Can you work these out from the model? Positions are in its coordinate system, mm. Face numbers are marked on the shaded views. Coordinates: 2 decimals unless noted, no trailing zeros. Order: outer loops, then holes, each group sorted by start corner. A loop starts at its lowest first (then second) coordinate and runs counter-clockwise, first axis right, second up. Notation, with made-up numbers: M 74,55.25 L 87,55.25 A31 ccw 87,88.25 Z; hole C -0.5,49 d1. An arc over 180 degrees is marked long. Answer as CSV lines item,"result". Start each with the question number.
1. Will these pins go through, and if not, where does the flat tip stop? pin 1 (1.6 mm diameter, centred on y = 2.54, z = 0, fed in from +X); pin 2 (10 mm diameter, centred on x = 11, y = 11, fed in from +Z); pin 3 (2 mm diameter, centred on y = 5, z = -1.5, fed in from +X).
2. If we mould it in two halves opening along X, with no side actions, what happens to the marked faces 1, 2 and 3? For each: released by +X, released by -X, zero draft, split by the parting line, or undercut.
3. I need wall thicknesses on line 1 along X through (y, z) = (8.25, 0); line 2 along Z through (x, y) = (4, 6.75). Which ranges of each line are inside material? Lowest first, please. Write a range as from..to.
4. If we section it at B-B (y = 5): List the corners of the cut face in (x, z) for me (1 decimal).
5. If we section it at A-A (x = 0): List the corners of the cut face in (y, z) for me (1 decimal).
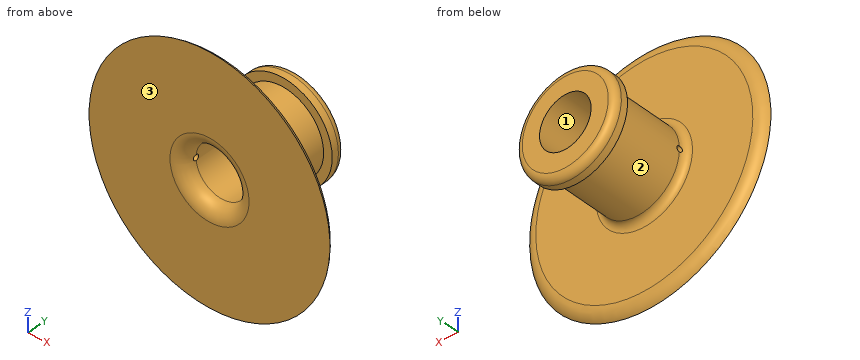
```python
from build123d import *

# Parameters (mm, degrees)
SKETCH1_R           = 22.225
BOSS_EXTRUDE1_DEPTH = 1.27
SKETCH2_R           = 7.62
BOSS_EXTRUDE2_DEPTH = 16.256
SKETCH3_R           = 4.7625
CUT_EXTRUDE1_DEPTH  = 36.986968836
FILLET1_R           = 1.27
SKETCH4_R           = 0.508
CUT_EXTRUDE2_DEPTH  = 36.986968836
FILLET2_R           = 2.54
FILLET3_R           = 2.54
SKETCH5_W           = 1.5875
SKETCH5_H           = 2.54
FILLET4_R           = 1.27


with BuildPart() as part:
    # Sketch1 → Boss-Extrude1 (new body)
    with BuildSketch(Plane(origin=(0, 0, 0), x_dir=(1, 0, 0), z_dir=(0, 1, 0))):
        with Locations(Location((0, 0, 0), (0, 0, 270))):
            Circle(SKETCH1_R)
    extrude(amount=BOSS_EXTRUDE1_DEPTH)

    # Sketch2 → Boss-Extrude2 (add)
    with BuildSketch(Plane(origin=(0, 1.27, 0), x_dir=(1, 0, 0), z_dir=(0, 1, 0))):
        with Locations(Location((0, 0, 0), (0, 0, 270))):
            Circle(SKETCH2_R)
    extrude(amount=BOSS_EXTRUDE2_DEPTH)

    # Sketch3 → Cut-Extrude1 (cut, through all)
    with BuildSketch(Plane(origin=(0, 17.526, 0), x_dir=(1, 0, 0), z_dir=(0, 1, 0))):
        with Locations(Location((0, 0, 0), (0, 0, 270))):
            Circle(SKETCH3_R)
    extrude(amount=-CUT_EXTRUDE1_DEPTH, mode=Mode.SUBTRACT)

    # Fillet1
    fillet1_edges = [part.edges().sort_by_distance(p)[0] for p in [
        (0, 1.27, -7.62),
    ]]
    fillet(fillet1_edges, radius=FILLET1_R)

    # Sketch4 → Cut-Extrude2 (cut, through all)
    with BuildSketch(Plane(origin=(0, 0, 0), x_dir=(0, 0, -1), z_dir=(1, 0, 0))):
        with Locations((0, 2.54)):
            Circle(SKETCH4_R)
    extrude(amount=-CUT_EXTRUDE2_DEPTH, mode=Mode.SUBTRACT)

    # Fillet2
    # the kernel refuses this fillet: 2.54 mm, written as the material it takes off along each edge
    with BuildSketch(Plane(origin=(0, 1.27, 0), x_dir=(0, 0, 1), z_dir=(-1, 0, 0))) as fillet2_piece_1:
        with BuildLine():
            CenterArc((20.025295474, -2.54), FILLET2_R, 30, 60)
            Line((22.225, -1.27), (22.268994091, -1.2446))
            ThreePointArc((22.268994091, -1.2446), (22.2758, -0.635), (22.2758, 0))
            Line((22.2758, 0), (22.225, 0.0508))
            Line((22.225, 0.0508), (20.025295474, 0.0508))
            Line((20.025295474, 0.0508), (20.025295474, 0))
        make_face()
    revolve(axis=Axis((0, 1.27, 0), (0, 1, 0)), mode=Mode.SUBTRACT)

    # Fillet3
    # the kernel refuses this fillet: 2.54 mm, written as the material it takes off along each edge
    with BuildSketch(Plane(origin=(0, 0, 0), x_dir=(0, 0, 1), z_dir=(-1, 0, 0))) as fillet3_piece_1:
        with BuildLine():
            CenterArc((4.7625 + FILLET3_R, FILLET3_R), FILLET3_R, 180, 90)
            Line((4.7625, FILLET3_R), (4.7625, 0))
            Line((4.7625, 0), (4.7625 + FILLET3_R, 0))
        make_face()
    revolve(axis=Axis((0, 0, 0), (0, 1, 0)), mode=Mode.SUBTRACT)

    # Sketch5 → Revolve1 (revolve)
    with BuildSketch(Plane.XY, mode=Mode.PRIVATE) as revolve1_sk:
        with Locations((8.41375, 16.256)):
            Rectangle(SKETCH5_W, SKETCH5_H)
    revolve(revolve1_sk.sketch.rotate(Axis((0, 19.916609625, 0), (0, -1, 0)), 183.822553729), axis=Axis((0, 19.916609625, 0), (0, -1, 0)))

    # Fillet4
    fillet4_edges = [part.edges().sort_by_distance(p)[0] for p in [
        (9.187016104, 17.526, 0.613833333),
    ]]
    fillet(fillet4_edges, radius=FILLET4_R)


solid = part.part
```
Solved:
1,pin 1,"x = 7.9"
1,pin 2,"z = 4.7"
1,pin 3,"x = 7.6"
2,face 1,"undercut"
2,face 2,"split by the parting line"
2,face 3,"zero draft"
3,line 1,"-7.62..-4.76, 4.76..7.62"
3,line 2,"-6.49..-2.58, 2.58..6.49"
4,outline,"C 0,0 d15.2; hole C 0,0 d9.5"
5,outline,"M 0,-22.2 A2.5 ccw 1.3,-20 L 1.3,-8.9 A1.3 cw 2.5,-7.6 L 15,-7.6 L 15,-9.2 L 16.3,-9.2 A1.3 ccw 17.5,-7.9 L 17.5,-4.8 L 2.5,-4.8 A2.5 ccw 0,-7.3 Z; M 0,7.3 A2.5 ccw 2.5,4.8 L 17.5,4.8 L 17.5,7.9 A1.3 ccw 16.3,9.2 L 15,9.2 L 15,7.6 L 2.5,7.6 A1.3 cw 1.3,8.9 L 1.3,20 A2.5 ccw 0,22.2 Z"
